Source: CAD feature listing. Evaluate the final solid. Frame: model axes, mm. A direction names the side the tool comes from. Give positions to 0.01 mm unless a question says otherwise; leave off trailing zeros. Order: outer loops, then holes, each group sorted by start corner. A loop starts at its lowest first (then second) coordinate and runs counter-clockwise, first axis right, second up. Notation, with made-up numbers: M 47,-17 L 68,-17 A25 ccw 68,14 Z; hole C -13,-29.5 d6. An arc over 180 degrees is marked long. Answer as a JSON object with one key per item and string values. Group by question number.
1. Pin query (flat end, axial travel): P1, Ø1.5, axis at y = -1, z = 23.5, coming from the +X side; P2, Ø1.6, axis at y = 0.5, z = 86.5, coming from the +X side; P3, Ø1.6, axis at y = 0, z = 85.5, coming from the -X side. Return the tip coordinate at first contact, or that it passes through.
2. Section query A-A (y = 0). Output: boundary loops of the cut face in (x, z), plus the area to 3 significant figures.
3. Set-up query: faces 1 (the flat face through (-2.4, 4.1, 80)), 2 (the flat face through (2.28, 3.88, 4.93)), 3 (the flat face through (4.5, 0, 85)). Return all of +Z, -Z, +X, -X, +Y, -Y with unobstructed straight access to the full face (end or side cutting, diameter ignored); none if empty.
4. Material intervals for L1, parallel to X at y = -1.5, z = 5.5; L2, parallel to X at y = -0.25, z = 67.5; L3, parallel to Y at x = -2, z = 32, sorted ascending. Write a range as [from, to].
5. Section query B-B (z = 69). Output: boundary loops of the cut face in (x, y), plus the area to 3 significant figures.
6. Section query C-C (x = 1). Output: boundary loops of the cut face in (y, z).
from build123d import *

# Parameters (mm, degrees)
SALIENTE_EXTRUIR1_DEPTH = 10
CROQUIS2_R              = 5.196152423
SALIENTE_EXTRUIR3_DEPTH = 70
SALIENTE_EXTRUIR4_DEPTH = 10


with BuildPart() as part:
    # Croquis1 → Saliente-Extruir1 (new body)
    with BuildSketch(Plane.XY):
        Polygon((0, 5.196152423), (-4.5, 2.598076211), (-4.5, -2.598076211), (0, -5.196152423), (4.5, -2.598076211), (4.5, 2.598076211), align=None)
    extrude(amount=SALIENTE_EXTRUIR1_DEPTH)

    # Croquis2 → Saliente-Extruir3 (add)
    with BuildSketch(Plane.XY.offset(10)):
        Circle(CROQUIS2_R)
    extrude(amount=SALIENTE_EXTRUIR3_DEPTH)

    # Croquis3 → Saliente-Extruir4 (add)
    with BuildSketch(Plane.XY.offset(80)):
        Polygon((0, 5.196152423), (-4.5, 2.598076211), (-4.5, -2.598076211), (0, -5.196152423), (4.5, -2.598076211), (4.5, 2.598076211), align=None)
    extrude(amount=SALIENTE_EXTRUIR4_DEPTH)


solid = part.part
Answer sheet:
{
 "1": {"P1": "x = 5.19", "P2": "x = 4.5", "P3": "x = -4.5"},
 "2": {"outline": "M -5.2,10 L -4.5,10 L -4.5,0 L 4.5,0 L 4.5,10 L 5.2,10 L 5.2,80 L 4.5,80 L 4.5,90 L -4.5,90 L -4.5,80 L -5.2,80 Z", "area": "907 mm^2"},
 "3": {"face 1": "+Z, -X, +Y", "face 2": "-Z, +X, +Y", "face 3": "+Z, +X, +Y, -Y"},
 "4": {"L1": "[-4.5, 4.5]", "L2": "[-5.19, 5.19]", "L3": "[-4.8, 4.8]"},
 "5": {"outline": "C 0,0 d10.39", "area": "84.8 mm^2"},
 "6": {"outline": "M -5.1,10 L -4.62,10 L -4.62,0 L 4.62,0 L 4.62,10 L 5.1,10 L 5.1,80 L 4.62,80 L 4.62,90 L -4.62,90 L -4.62,80 L -5.1,80 Z"}
}
